The model under review builds one solid part; all positions refer to its coordinate system, in mm. A direction names the side the tool comes from. Give positions to 0.01 mm unless a question says otherwise; leave off trailing zeros. Order: outer loops, then holes, each group sorted by start corner. A loop starts at its lowest first (then second) coordinate and runs counter-clockwise, first axis right, second up. Notation, with made-up numbers: (-4, -1) - (7, -1) arc R28 ccw to (7, 36) - close; hole circle Ø11 at (4.5, -31.75). An arc over 180 degrees is marked (long way). Write item = value, one per line. Start each with the question number.
1. We need section D-D, the plane z = -46. Give the boundary of the cut face in (x, y) (3 decimals), and give its area (3 significant figures).
2. For P1, Ø5.5, axis at x = 3.48, z = -30.2, coming from the -Y side; P2, Ø1.6, axis at x = -17.5, y = 1, coming from the -Z side; P3, Ø1, axis at y = 1, z = -53.5, coming from the +X side, all flat-tipped, find the tip position at first contact; note any pin that passes through.
3. Machinability: for faces 1 (the flat face through (-9.219, 2, -43)), 2 (the flat face through (4, 0, -22)), 3 (the flat face through (29, 2, -17.496)), which of the approach directions +Z, -Z, +X, -X, +Y, -Y give a long, thin tool a straight path to every point of the face, cutting with its end or side? Answer none if there is none.
4. We need section C-C, the plane y = 2. Give the boundary of the cut face in (x, z).
5. We need section A-A, the plane x = 4. Give the boundary of the cut face in (y, z) (3 decimals), and give its area (3 significant figures).
6. Mouldability with a two-part tool opening along X and no side actions: class faces 4 (the cylindrical face through (-19.648, 1.565, -5.511)), 5 (the cylindrical face through (-33.895, 1.565, -16.732)), 6 (the cylindrical face through (15.42, 1.57, -67.57)), 7 (the flat face through (4, 2, 7.904)) as pulls with the +X half, pulls with the -X half, needs draft (parallel to the pull), parting line crosses it, or undercut.
7. We need section B-B, the plane x = 29. Give the boundary of the cut face in (y, z) (3 decimals), and give its area (3 significant figures).
8. Wall thickness on probe 1 along X at (y, z) = (1.5, -33); probe 2 along Z at (x, y) = (25, 0.3); probe 3 along X at (y, z) = (0.2, -55.5): over which ranges is each line inside the solid? List them lowest first.
from build123d import *

# Parameters (mm, degrees)
SKETCH1_R           = 2.38125
BOSS_EXTRUDE1_DEPTH = 3.175


with BuildPart() as part:
    # Sketch1 → Boss-Extrude1 (new body)
    with BuildSketch(Plane(origin=(0, 0, 0), x_dir=(1, 0, 0), z_dir=(0, 1, 0))):
        with BuildLine():
            Line((18.720543933, 17.495711297), (39.040543933, 17.495711297))
            ThreePointArc((39.040543933, 17.495711297), (40.836595157, 16.751762521), (41.580543933, 14.955711297))
            Line((41.580543933, 14.955711297), (41.580543933, -5.364288703))
            ThreePointArc((41.580543933, -5.364288703), (40.836595157, -7.160339927), (39.040543933, -7.904288703))
            Line((39.040543933, -7.904288703), (-32.079456067, -7.904288703))
            ThreePointArc((-32.079456067, -7.904288703), (-33.875507291, -7.160339927), (-34.619456067, -5.364288703))
            Line((-34.619456067, -5.364288703), (-34.619456067, 14.955711297))
            ThreePointArc((-34.619456067, 14.955711297), (-33.875507291, 16.751762521), (-32.079456067, 17.495711297))
            Line((-32.079456067, 17.495711297), (-11.759456067, 17.495711297))
            ThreePointArc((-11.759456067, 17.495711297), (-9.963404843, 18.239660073), (-9.219456067, 20.035711297))
            Line((-9.219456067, 20.035711297), (-9.219456067, 65.755711297))
            ThreePointArc((-9.219456067, 65.755711297), (-8.475507291, 67.551762521), (-6.679456067, 68.295711297))
            Line((-6.679456067, 68.295711297), (13.640543933, 68.295711297))
            ThreePointArc((13.640543933, 68.295711297), (15.436595157, 67.551762521), (16.180543933, 65.755711297))
            Line((16.180543933, 65.755711297), (16.180543933, 20.035711297))
            ThreePointArc((16.180543933, 20.035711297), (16.924492709, 18.239660073), (18.720543933, 17.495711297))
        make_face()
        with Locations((3.480543933, 4.795711297)):
            Circle(SKETCH1_R, mode=Mode.SUBTRACT)
        with Locations((-21.919456067, 4.795711297)):
            Circle(SKETCH1_R, mode=Mode.SUBTRACT)
        with Locations((28.880543933, 4.795711297)):
            Circle(SKETCH1_R, mode=Mode.SUBTRACT)
        with Locations((3.480543933, 30.195711297)):
            Circle(SKETCH1_R, mode=Mode.SUBTRACT)
        with Locations((3.480543933, 55.595711297)):
            Circle(SKETCH1_R, mode=Mode.SUBTRACT)
    extrude(amount=BOSS_EXTRUDE1_DEPTH)


solid = part.part
Model answer:
q1.outline = (-9.219, 0) - (16.181, 0) - (16.181, 3.175) - (-9.219, 3.175) - close
q1.area = 80.6 mm2
q2.P1 = 0
q2.P2 = -17.5
q2.P3 = 16.18
q3.face_1 = -Z, -X, +Y, -Y
q3.face_2 = +Z, -Z, +X, -X, -Y
q3.face_3 = -Z, +X, +Y, -Y
q4.outline = (-34.62, -14.96) arc R2.54 ccw to (-32.08, -17.5) - (-11.76, -17.5) arc R2.54 cw to (-9.22, -20.04) - (-9.22, -65.76) arc R2.54 ccw to (-6.68, -68.3) - (13.64, -68.3) arc R2.54 ccw to (16.18, -65.76) - (16.18, -20.04) arc R2.54 cw to (18.72, -17.5) - (39.04, -17.5) arc R2.54 ccw to (41.58, -14.96) - (41.58, 5.36) arc R2.54 ccw to (39.04, 7.9) - (-32.08, 7.9) arc R2.54 ccw to (-34.62, 5.36) - close; hole circle Ø4.76 at (-21.92, -4.8); hole circle Ø4.76 at (3.48, -55.6); hole circle Ø4.76 at (3.48, -30.2); hole circle Ø4.76 at (3.48, -4.8); hole circle Ø4.76 at (28.88, -4.8)
q5.outline = (0, -68.296) - (3.175, -68.296) - (3.175, -57.92) - (0, -57.92) - close; (0, -53.272) - (3.175, -53.272) - (3.175, -32.52) - (0, -32.52) - close; (0, -27.872) - (3.175, -27.872) - (3.175, -7.12) - (0, -7.12) - close; (0, -2.472) - (3.175, -2.472) - (3.175, 7.904) - (0, 7.904) - close
q5.area = 198 mm2
q6.face_4 = undercut
q6.face_5 = pulls with the -X half
q6.face_6 = pulls with the +X half
q6.face_7 = needs draft
q7.outline = (0, -17.496) - (3.175, -17.496) - (3.175, -7.174) - (0, -7.174) - close; (0, -2.417) - (3.175, -2.417) - (3.175, 7.904) - (0, 7.904) - close
q7.area = 65.5 mm2
q8.probe_1 = -9.22 to 16.18
q8.probe_2 = -17.5 to 7.9
q8.probe_3 = -9.22 to 1.1, 5.86 to 16.18
